The model under review builds one solid part; all positions refer to its coordinate system, in mm. Coordinates: 2 decimals unless noted, no trailing zeros. Order: outer loops, then holes, each group sorted by start corner. A loop starts at its lowest first (then second) coordinate and runs counter-clockwise, first axis right, second up. Notation, with made-up numbers: (-35.75, 6) -> (9.25, 6) arc R19 cw to (9.25, 29) -> close; hole circle Ø10 at (85, 85). An arc over 180 degrees is marked (long way). Use one line per item in the form item = value.
from build123d import *

# Parameters (mm, degrees)
SKETCH001_R             = 2.1
SKETCH001_R_2           = 1
SKETCH001_R_3           = 1.55
SKETCH001_R_4           = 1.5
PAD001_DEPTH            = 3
BODY001_PLACEMENT_ANGLE = 180
SKETCH_R                = 2.1
SKETCH_R_2              = 1
SKETCH_R_3              = 1.55
SKETCH_R_4              = 1.5
PAD_DEPTH               = 3


with BuildPart() as body001:
    # Sketch001 → Pad001 (new body)
    with BuildSketch(Plane.XY):
        with BuildLine():
            ThreePointArc((59.929397, -17.053147), (73.5, 0), (59.929397, 17.053147))
            ThreePointArc((51.751169, 46.191946), (50.930057, 30.24442), (59.929397, 17.053147))
            ThreePointArc((51.751169, 46.191946), (49.522386, 75.284598), (23.602068, 61.88732))
            ThreePointArc((0, 48), (13.692291, 51.729393), (23.602068, 61.88732))
            Line((0, 48), (0, -48))
            ThreePointArc((23.602068, -61.88732), (13.692291, -51.729393), (0, -48))
            ThreePointArc((23.602068, -61.88732), (49.522386, -75.284598), (51.751169, -46.191946))
            ThreePointArc((59.929397, -17.053147), (50.930057, -30.24442), (51.751169, -46.191946))
        make_face()
        with Locations((41, 60)):
            Circle(SKETCH001_R, mode=Mode.SUBTRACT)
        with Locations((56, 0)):
            Circle(SKETCH001_R, mode=Mode.SUBTRACT)
        with Locations((41, -60)):
            Circle(SKETCH001_R, mode=Mode.SUBTRACT)
        with Locations((41, 71)):
            Circle(SKETCH001_R_2, mode=Mode.SUBTRACT)
        with Locations((41, 49)):
            Circle(SKETCH001_R_2, mode=Mode.SUBTRACT)
        with Locations((52, 60)):
            Circle(SKETCH001_R_2, mode=Mode.SUBTRACT)
        with Locations((30, 60)):
            Circle(SKETCH001_R_2, mode=Mode.SUBTRACT)
        with Locations((56, 11)):
            Circle(SKETCH001_R_2, mode=Mode.SUBTRACT)
        with Locations((56, -11)):
            Circle(SKETCH001_R_2, mode=Mode.SUBTRACT)
        with Locations((67, 0)):
            Circle(SKETCH001_R_2, mode=Mode.SUBTRACT)
        with Locations((45, 0)):
            Circle(SKETCH001_R_2, mode=Mode.SUBTRACT)
        with Locations((41, -49)):
            Circle(SKETCH001_R_2, mode=Mode.SUBTRACT)
        with Locations((41, -71)):
            Circle(SKETCH001_R_2, mode=Mode.SUBTRACT)
        with Locations((52, -60)):
            Circle(SKETCH001_R_2, mode=Mode.SUBTRACT)
        with Locations((30, -60)):
            Circle(SKETCH001_R_2, mode=Mode.SUBTRACT)
        with Locations((8, -42)):
            Circle(SKETCH001_R_3, mode=Mode.SUBTRACT)
        with Locations((8, -30)):
            Circle(SKETCH001_R_3, mode=Mode.SUBTRACT)
        with Locations((8, 30)):
            Circle(SKETCH001_R_3, mode=Mode.SUBTRACT)
        with Locations((8, 42)):
            Circle(SKETCH001_R_3, mode=Mode.SUBTRACT)
        with Locations((26, 17.5)):
            Circle(SKETCH001_R_4, mode=Mode.SUBTRACT)
        with Locations((26, -17.5)):
            Circle(SKETCH001_R_4, mode=Mode.SUBTRACT)
    extrude(amount=PAD001_DEPTH)


with BuildPart() as body001_1:
    # Body001 placement: moved
    add(body001.part.rotate(Axis((0, 0, 0), (0, 0, 1)), BODY001_PLACEMENT_ANGLE))


with BuildPart() as fusion:
    # Sketch → Pad (new body)
    with BuildSketch(Plane.XY):
        with BuildLine():
            ThreePointArc((59.929397, -17.053147), (73.5, 0), (59.929397, 17.053147))
            ThreePointArc((51.751169, 46.191946), (50.930057, 30.24442), (59.929397, 17.053147))
            ThreePointArc((51.751169, 46.191946), (49.522386, 75.284598), (23.602068, 61.88732))
            ThreePointArc((0, 48), (13.692291, 51.729393), (23.602068, 61.88732))
            Line((0, 48), (0, -48))
            ThreePointArc((23.602068, -61.88732), (13.692291, -51.729393), (0, -48))
            ThreePointArc((23.602068, -61.88732), (49.522386, -75.284598), (51.751169, -46.191946))
            ThreePointArc((59.929397, -17.053147), (50.930057, -30.24442), (51.751169, -46.191946))
        make_face()
        with Locations((41, 60)):
            Circle(SKETCH_R, mode=Mode.SUBTRACT)
        with Locations((56, 0)):
            Circle(SKETCH_R, mode=Mode.SUBTRACT)
        with Locations((41, -60)):
            Circle(SKETCH_R, mode=Mode.SUBTRACT)
        with Locations((41, 71)):
            Circle(SKETCH_R_2, mode=Mode.SUBTRACT)
        with Locations((41, 49)):
            Circle(SKETCH_R_2, mode=Mode.SUBTRACT)
        with Locations((52, 60)):
            Circle(SKETCH_R_2, mode=Mode.SUBTRACT)
        with Locations((30, 60)):
            Circle(SKETCH_R_2, mode=Mode.SUBTRACT)
        with Locations((56, 11)):
            Circle(SKETCH_R_2, mode=Mode.SUBTRACT)
        with Locations((56, -11)):
            Circle(SKETCH_R_2, mode=Mode.SUBTRACT)
        with Locations((67, 0)):
            Circle(SKETCH_R_2, mode=Mode.SUBTRACT)
        with Locations((45, 0)):
            Circle(SKETCH_R_2, mode=Mode.SUBTRACT)
        with Locations((41, -49)):
            Circle(SKETCH_R_2, mode=Mode.SUBTRACT)
        with Locations((41, -71)):
            Circle(SKETCH_R_2, mode=Mode.SUBTRACT)
        with Locations((52, -60)):
            Circle(SKETCH_R_2, mode=Mode.SUBTRACT)
        with Locations((30, -60)):
            Circle(SKETCH_R_2, mode=Mode.SUBTRACT)
        with Locations((8, -42)):
            Circle(SKETCH_R_3, mode=Mode.SUBTRACT)
        with Locations((8, -30)):
            Circle(SKETCH_R_3, mode=Mode.SUBTRACT)
        with Locations((8, 30)):
            Circle(SKETCH_R_3, mode=Mode.SUBTRACT)
        with Locations((8, 42)):
            Circle(SKETCH_R_3, mode=Mode.SUBTRACT)
        with Locations((26, 17.5)):
            Circle(SKETCH_R_4, mode=Mode.SUBTRACT)
        with Locations((26, -17.5)):
            Circle(SKETCH_R_4, mode=Mode.SUBTRACT)
    extrude(amount=PAD_DEPTH)

    # Fusion: union Body001
    add(body001_1.part)


solid = fusion.part
Item 1: Clearance check with flat-ended pins moving along their axes: pin 1 (1.8 mm diameter, centred on x = -41, y = -71, fed in from +Z); pin 2 (1.5 mm diameter, centred on x = -56.5, z = 0.5, fed in from -Y). State where each tip first meets the part, or that it passes through.
Results found:
pin_1 = through
pin_2 = -69.42
Item 2: We need section B-B (y = 37.5). Write out the cut boundary in (x, z) (3 decimals), plus the area to 3 significant figures.
Results found:
outline = (-50.005, 0) -> (50.005, 0) -> (50.005, 3) -> (-50.005, 3) -> close
area = 300 mm²
Item 3: We need section C-C (z = 1.5). State how many separate pieces and enclosed holes the cut face has, plus the area to 3 significant figures.
Results found:
separate_pieces = 1
enclosed_holes = 42
area = 14,900 mm²
Item 4: We need section A-A (x = 48). Write out the cut boundary in (y, z), plus the area to 3 significant figures.
Results found:
outline = (-76.04, 0) -> (76.04, 0) -> (76.04, 3) -> (-76.04, 3) -> close
area = 456 mm²
Item 5: Draft analysis for pull direction Y (two halves, no side actions). For faces 1 (the face through (73.497, -0.329, 1.479)), 2 (the face through (-51, 30, 1)), 3 (the face through (1, -1, 0)), state which applies: released by +Y, released by -Y, zero draft, split by the parting line, or undercut.
Results found:
face_1 = split by the parting line
face_2 = undercut
face_3 = zero draft
Item 6: To check wall thickness, follow L1, parallel to Y at x = -8, z = 1.8; L2, parallel to Y at x = 52, z = 1.25; L3, parallel to Y at x = -56, z = 1.1. State the ranges of each line that lie inside material, in increasing order. Write a range as from..to.
Results found:
L1 = -49.21..-43.55, -40.45..-31.55, -28.45..28.45, 31.55..40.45, 43.55..49.21
L2 = -73.61..-61, -59..-46.39, -27.2..27.2, 46.39..59, 61..73.61
L3 = -69.01..-50.99, -20.75..-12, -10..-2.1, 2.1..10, 12..20.75, 50.99..69.01
